```python
from build123d import *

# Parameters (mm, degrees)
EXTRUDE_THIN1_DEPTH = 279.4
FILLET1_R           = 1.016


with BuildPart() as part:
    # Sketch1 → Extrude-Thin1 (new body)
    with BuildSketch(Plane.XY):
        with BuildLine():
            Line((0, 4.7625), (0, 0))
            Line((0, 0), (-6.35, 0))
            Line((-6.35, 0), (-6.35, 5.55625))
            Line((-6.35, 5.55625), (-9.525, 5.55625))
            ThreePointArc((-9.525, 5.55625), (-12.547291902, 12.852708098), (-19.84375, 15.875))
            Line((-19.84375, 15.875), (-19.84375, 19.84375))
            Line((-19.84375, 19.84375), (-25.4, 19.84375))
            Line((-25.4, 19.84375), (-25.4, 32.54375))
            Line((-25.4, 32.54375), (-22.225, 32.54375))
            Line((-22.225, 32.54375), (-22.225, 31.52775))
            Line((-22.225, 31.52775), (-24.384, 31.52775))
            Line((-24.384, 31.52775), (-24.384, 20.85975))
            Line((-24.384, 20.85975), (-18.82775, 20.85975))
            Line((-18.82775, 20.85975), (-18.82775, 16.845373153))
            ThreePointArc((-18.82775, 16.845373153), (-11.828871412, 13.571128588), (-8.554626847, 6.57225))
            Line((-8.554626847, 6.57225), (-5.334, 6.57225))
            Line((-5.334, 6.57225), (-5.334, 1.016))
            Line((-5.334, 1.016), (-1.016, 1.016))
            Line((-1.016, 1.016), (-1.016, 4.7625))
            Line((-1.016, 4.7625), (0, 4.7625))
        make_face()
    extrude(amount=-EXTRUDE_THIN1_DEPTH)

    # Fillet1
    fillet1_edges = [part.edges().sort_by_distance(p)[0] for p in [
        (-18.82775, 20.85975, -139.7),
        (-5.334, 6.57225, -139.7),
        (0, 0, -139.7),
        (-6.35, 0, -139.7),
        (-9.525, 5.55625, -139.7),
        (-19.84375, 15.875, -139.7),
        (-25.4, 19.84375, -139.7),
        (-25.4, 32.54375, -139.7),
    ]]
    fillet(fillet1_edges, radius=FILLET1_R)


solid = part.part
```
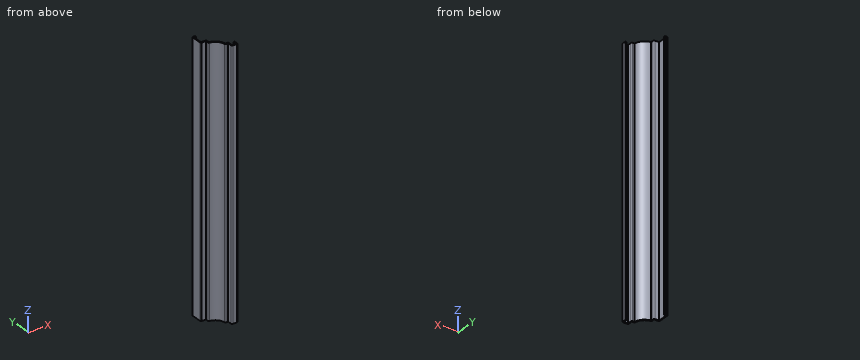
For this review, take the finished solid that the model builds, in its own axes (mm). Coordinates: 2 decimals unless noted, no trailing zeros. Order: outer loops, then holes, each group sorted by start corner. A loop starts at its lowest first (then second) coordinate and runs counter-clockwise, first axis right, second up. Notation, with made-up numbers: (-37, 43) -> (-5, 43) arc R30 ccw to (-5, 71) -> close; hole circle Ø7 at (-40, 70.25). An arc over 180 degrees is marked (long way). Use CSV: the item, a comma, the result in double quotes. Start each with the question number.
Item 1: We need section C-C, the plane x = -13.5. Give the boundary of the cut face in (y, z), then the cut area to 3 significant figures.
Item 2: Insertion check: pin 1 (1.4 mm diameter, centred on y = 3.5, z = -193.5, fed in from -X); pin 2 (1.5 mm diameter, centred on x = -4.5, z = -199, fed in from -Y); pin 3 (1.1 mm diameter, centred on x = -7.5, z = -118, fed in from -Y); pin 4 (3.5 mm diameter, centred on y = 18, z = -144.5, fed in from -X). Each pin has a flat end and moves straight along its axis. Give the tip position at first contact, or say it passes through.
Item 3: Wall thickness on probe 1 along X at (y, z) = (5.5, -34.5); probe 2 along X at (y, z) = (2, -87); probe 3 along Y at (x, z) = (-20, -31): over which ranges is each line inside the solid? List them lowest first.
Item 4: We need section B-B, the plane y = 26. Give the boundary of the cut face in (x, z), then the cut area to 3 significant figures.
Derived:
1,outline,"(13.69, -279.4) -> (14.95, -279.4) -> (14.95, 0) -> (13.69, 0) -> close"
1,area,"351 mm^2"
2,pin 1,"stops at x = -6.35"
2,pin 2,"stops at y = 0"
2,pin 3,"stops at y = 5.56"
2,pin 4,"stops at x = -19.84"
3,probe 1,"x = -6.35 to -5.33"
3,probe 2,"x = -6.35 to -5.33, -1.02 to 0"
3,probe 3,"y = 19.84 to 20.86"
4,outline,"(-25.4, -279.4) -> (-24.38, -279.4) -> (-24.38, 0) -> (-25.4, 0) -> close"
4,area,"284 mm^2"
